The model under review builds one solid part; all positions refer to its coordinate system, in mm. A direction names the side the tool comes from. Round coordinates to 2 decimals unless told otherwise and drop trailing zeros. Loops run counter-clockwise (first coordinate to the right, second up) from the corner with the lowest first, then second, coordinate; pieces in that order, holes last. Notation, with made-up numbers: M -10.75,43.25 L 18.25,43.25 A23 cw 18.25,73.25 Z; hole C -14,89.5 d1. An arc over 180 degrees is marked long. One line per question, with ' | ' between items.
from build123d import *

# Parameters (mm, degrees)
F1_DEPTH = 38
F2_R     = 1.25
F2_R_2   = 1.5
F3_DEPTH = 4
F4_R     = 2
F5_DEPTH = 2


with BuildPart() as f1:
    # F0 (on Right) → F1 (new body)
    with BuildSketch(Plane.YZ):
        Polygon((0, 26), (0, 0), (20, 0), (20, 4), (55, 4), (55, 0), (75, 0), (75, 26), align=None)
    extrude(amount=F1_DEPTH)

    # F2 (on face) → F3 (cut)
    with BuildSketch(Plane.XY.offset(26)):
        with BuildLine():
            Line((18.5, 34.5419601085), (18.5, 40.4580398915))
            ThreePointArc((18.5, 40.4580398915), (16, 37.5), (18.5, 34.5419601085))
        make_face()
        with BuildLine():
            Line((19.5, 34.5419601085), (19.5, 40.4580398915))
            ThreePointArc((19.5, 40.4580398915), (19, 40.5), (18.5, 40.4580398915))
            Line((18.5, 40.4580398915), (18.5, 34.5419601085))
            ThreePointArc((18.5, 34.5419601085), (19, 34.5), (19.5, 34.5419601085))
        make_face()
        with BuildLine():
            ThreePointArc((19.5, 34.5419601085), (21.2912878475, 35.5635083269), (22, 37.5))
            ThreePointArc((22, 37.5), (21.2912878475, 39.4364916731), (19.5, 40.4580398915))
            Line((19.5, 40.4580398915), (19.5, 34.5419601085))
        make_face()
        with BuildLine():
            Line((19.5, 34.25), (19.5, 34.5419601085))
            ThreePointArc((19.5, 34.5419601085), (19, 34.5), (18.5, 34.5419601085))
            Line((18.5, 34.5419601085), (18.5, 34.25))
            Line((18.5, 34.25), (19.5, 34.25))
        make_face()
        with Locations((19, 43.5)):
            Circle(F2_R)
        with Locations((35, 37.5)):
            Circle(F2_R_2)
        with Locations((3, 37.5)):
            Circle(F2_R_2)
        with Locations((15.7561550967, 42.5475211979)):
            Circle(F2_R)
        with Locations((13.5422080293, 39.9924900812)):
            Circle(F2_R)
        with Locations((13.061071348, 36.6461109755)):
            Circle(F2_R)
        with Locations((14.4655025493, 33.5708356016)):
            Circle(F2_R)
        with Locations((17.3096046506, 31.7430421608)):
            Circle(F2_R)
        with Locations((20.6903953311, 31.7430421554)):
            Circle(F2_R)
        with Locations((23.5344974382, 33.5708355872)):
            Circle(F2_R)
        with Locations((24.9389286493, 36.6461109566)):
            Circle(F2_R)
        with Locations((24.4577919786, 39.9924900638)):
            Circle(F2_R)
        with Locations((22.2438449193, 42.5475211876)):
            Circle(F2_R)
    extrude(amount=-F3_DEPTH, mode=Mode.SUBTRACT)

    # F4 (on face) → F5 (cut)
    with BuildSketch(Plane.XY.offset(26)):
        with Locations((5.1111, 71.5)):
            Circle(F4_R)
        with Locations((10.66665, 71.5)):
            Circle(F4_R)
        with Locations((16.2222, 71.5)):
            Circle(F4_R)
        with Locations((21.77775, 71.5)):
            Circle(F4_R)
        with Locations((27.3333, 71.5)):
            Circle(F4_R)
        with Locations((32.88885, 71.5)):
            Circle(F4_R)
        with Locations((5.1111, 3.5)):
            Circle(F4_R)
        with Locations((10.66665, 3.5)):
            Circle(F4_R)
        with Locations((16.2222, 3.5)):
            Circle(F4_R)
        with Locations((21.77775, 3.5)):
            Circle(F4_R)
        with Locations((27.3333, 3.5)):
            Circle(F4_R)
        with Locations((32.88885, 3.5)):
            Circle(F4_R)
    extrude(amount=-F5_DEPTH, mode=Mode.SUBTRACT)


solid = f1.part
1) Machinability: for faces 5 (the flat face through (14, 40, 22)), 6 (the flat face through (19, 0, 13)), which of the approach directions +Z, -Z, +X, -X, +Y, -Y give a long, thin tool a straight path to every point of the face, cutting with its end or side? Answer none if there is none.
Output values:
face 5: +Z | face 6: +Z, -Z, +X, -X, -Y
2) Add section A-A on y = 71.5. State the section outline as (x, z) points, then the cut area to 3 significant figures.
Output values:
outline: M 0,0 L 38,0 L 38,26 L 34.89,26 L 34.89,24 L 30.89,24 L 30.89,26 L 29.33,26 L 29.33,24 L 25.33,24 L 25.33,26 L 23.78,26 L 23.78,24 L 19.78,24 L 19.78,26 L 18.22,26 L 18.22,24 L 14.22,24 L 14.22,26 L 12.67,26 L 12.67,24 L 8.67,24 L 8.67,26 L 7.11,26 L 7.11,24 L 3.11,24 L 3.11,26 L 0,26 Z | area: 940 mm²
3) Mouldability with a two-part tool opening along X and no side actions: class faces 1 (the flat face through (19, 20, 2)), 2 (the flat face through (0, 37, 13)), 3 (the cylindrical face through (4.851, 73.483, 25.014)), 4 (the flat face through (5, 72, 24)) as +X half, -X half, draft (parallel to the pull), parting line (faces both ways), or undercut.
Output values:
face 1: draft | face 2: -X half | face 3: undercut | face 4: undercut
4) For line 1 (Z direction, x = 34, y = 42.5), list the stretches that pass through material, from the lowest coordinate up.
Output values:
line 1: z = 4 to 26
5) Insertion check: P1, Ø2, axis at x = 19, y = 43.5, coming from the +Z side; P2, Ø1, axis at x = 16.5, y = 32, coming from the -Z side. Each pin has a flat end and moves straight along its axis. Give the tip position at first contact, or say it passes through.
Output values:
P1: stops at z = 22 | P2: stops at z = 4
